Print and shaded views of the part. All mm, measured from the part's lowest x, y and z. Give positions to 0.01 mm unless a question says otherwise; leave off trailing zeros. Loops run counter-clockwise (first coordinate to the right, second up) from the corner with the lowest first, then second, coordinate; pieces in that order, holes last.
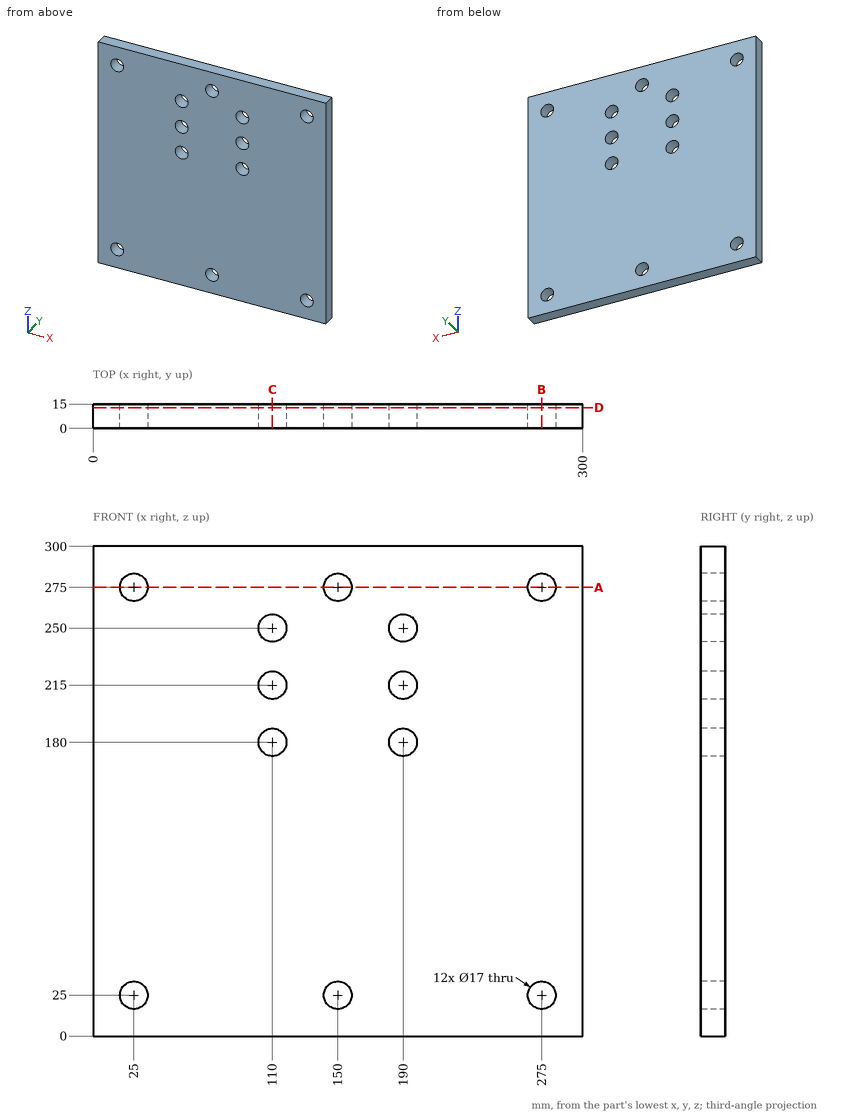
1. Saw through at D-D, the plane y = 12.75. Count the separate pieces of the cut face and the enclosed holes in it, and give its area (3 significant figures).
Responses:
separate pieces: 1
enclosed holes: 12
area: 87,300 mm2
2. Probe line 1 along Z through (x, y) = (25, 8.5); line 2 along Z through (x, y) = (190, 4.75); line 3 along Z through (x, y) = (145, 14.5). List the from-to ranges inside material, lowest first.
Responses:
line 1: z = 0 to 16.5, 33.5 to 266.5, 283.5 to 300
line 2: z = 0 to 171.5, 188.5 to 206.5, 223.5 to 241.5, 258.5 to 300
line 3: z = 0 to 18.13, 31.87 to 268.13, 281.87 to 300
3. Saw through at A-A, the plane z = 275. List the corners of the cut face in (x, y).
Responses:
outline: (0, 0) - (16.5, 0) - (16.5, 15) - (0, 15) - close; (33.5, 0) - (141.5, 0) - (141.5, 15) - (33.5, 15) - close; (158.5, 0) - (266.5, 0) - (266.5, 15) - (158.5, 15) - close; (283.5, 0) - (300, 0) - (300, 15) - (283.5, 15) - close
4. Saw through at B-B, the plane x = 275. List the corners of the cut face in (y, z), and give its area (3 significant figures).
Responses:
outline: (0, 0) - (15, 0) - (15, 16.5) - (0, 16.5) - close; (0, 33.5) - (15, 33.5) - (15, 266.5) - (0, 266.5) - close; (0, 283.5) - (15, 283.5) - (15, 300) - (0, 300) - close
area: 3,990 mm2
5. Saw through at C-C, the plane x = 110. List the corners of the cut face in (y, z), and give its area (4 significant figures).
Responses:
outline: (0, 0) - (15, 0) - (15, 171.5) - (0, 171.5) - close; (0, 188.5) - (15, 188.5) - (15, 206.5) - (0, 206.5) - close; (0, 223.5) - (15, 223.5) - (15, 241.5) - (0, 241.5) - close; (0, 258.5) - (15, 258.5) - (15, 300) - (0, 300) - close
area: 3,735 mm2
6. Drop a flat-ended pin along its axis: pin 1 (13.5 mm diameter, centred on x = 275, z = 275, fed in from +Y). Give the stop position or say it passes through.
Responses:
pin 1: passes through
